Geometry: final body of the model. Coordinates: model frame, mm. A direction names the side the tool comes from. Give positions to 0.01 mm unless a question says otherwise; leave off trailing zeros. Write each loop counter-clockwise with the first axis right and the second up, starting at its lowest first coordinate (ties: lowest second). Pieces come first, ordered by that corner, then holes.
Q1. Line query: line 1 (Y direction, x = 0, z = 48.5); line 2 (X direction, y = -0.5, z = 54); line 3 (Z direction, x = -2, y = -1.5). Output: solid intervals per line, ascending.
Q2. Reachability of faces 4 (the flat face through (0, 0, 1.8)), 5 (the cylindrical face through (-4.336, -19.524, 41.961)), 6 (the flat face through (6.5, -3.86, 1)) from +Z, -Z, +X, -X, +Y, -Y: full face, straight path, thin tool, end or side. Return the list, or none.
Q3. Mould query, pull axis X, two halves, no side actions, for faces 1 (the cylindrical face through (-14.985, 0.66, 39.318)), 2 (the conical face through (15.446, 4.864, 0.194)), 3 (the flat face through (18, -6, 81)). Classes: +X half, -X half, draft (parallel to the pull), parting line (faces both ways), or undercut.
Q4. Pin query (flat end, axial travel): pin 1 Ø4 at (x, y) = (-14, -9.5) entering from -Z; pin 2 Ø12 at (x, z) = (-10.5, 60) entering from +Y; pin 3 Ø0.5 at (y, z) = (6, 0.5) entering from +X; pin 4 Ø10 at (y, z) = (-11, 46) entering from +X. Return the tip coordinate at first contact, or that it passes through.
Q5. Section A-A (z = 70). Return the cut outline in (x, y).
from build123d import *

# Parameters (mm, degrees)
F0_R      = 20
F1_DEPTH  = 81
F2_R      = 18.432207
F3_DEPTH  = 5.2
F4_R      = 15
F5_DEPTH  = 74
F6_SIZE   = 4
F7_R      = 1.125396
F8_DEPTH  = 1
F10_DEPTH = 1


with BuildPart() as f1:
    # F0 (on Top) → F1 (new body)
    with BuildSketch(Plane.XY):
        Circle(F0_R)
    extrude(amount=F1_DEPTH)

    # F2 (on face) → F3 (cut)
    with BuildSketch(Plane.XY.offset(81)):
        Circle(F2_R)
    extrude(amount=-F3_DEPTH, mode=Mode.SUBTRACT)

    # F4 (on face) → F5 (cut)
    with BuildSketch(Plane.XY.offset(75.8)):
        Circle(F4_R)
    extrude(amount=-F5_DEPTH, mode=Mode.SUBTRACT)

    # F6
    f6_edges = [f1.edges().sort_by_distance(p)[0] for p in [
        (-20, 0, 0),
    ]]
    chamfer(f6_edges, length=F6_SIZE)

    # F7 (on face) → F8 (cut)
    with BuildSketch(Plane(origin=(0, 0, 0), x_dir=(1, 0, 0), z_dir=(0, 0, -1))):
        Polygon((-6.869866, 12.288648), (-8.467419, 8.024589), (-3.123957, -5.726644), (0.010684, -5.726644), align=None)
        with Locations((-8.475489, -0.289656)):
            Circle(F7_R)
        Polygon((-11.636892, -2.851509), (-13.690377, -5.736166), (-10.554273, -5.736166), align=None)
    extrude(amount=-F8_DEPTH, mode=Mode.SUBTRACT)

    # F9 (on face) → F10 (cut)
    with BuildSketch(Plane(origin=(0, 0, 0), x_dir=(1, 0, 0), z_dir=(0, 0, -1))):
        with BuildLine():
            Line((5.370924, 12.654014), (-2.24095, 12.654014))
            Line((-2.24095, 12.654014), (-2.24095, 11.971393))
            Line((-2.24095, 11.971393), (5.390103, 11.971393))
            ThreePointArc((5.390103, 11.971393), (8.507735, 8.271818), (6.310662, 3.961442))
            Line((6.310662, 3.961442), (4.144951, 3.961442))
            Line((4.144951, 3.961442), (4.144951, 3.490261))
            Line((4.144951, 3.490261), (6.310662, 3.490261))
            ThreePointArc((6.310662, 3.490261), (9.895604, -0.9064), (7.034451, -5.804997))
            Line((7.034451, -5.804997), (6.007162, -5.804997))
            Line((6.007162, -5.804997), (6.007162, -6.437175))
            Line((6.007162, -6.437175), (7.073962, -6.437175))
            ThreePointArc((7.073962, -6.437175), (10.562571, -1.134228), (6.777628, 3.961442))
            ThreePointArc((6.777628, 3.961442), (9.053097, 8.789785), (5.370924, 12.654014))
        make_face()
    extrude(amount=-F10_DEPTH, mode=Mode.SUBTRACT)


solid = f1.part
Computed:
1. line 1: y = -20 to -15, 15 to 20
1. line 2: x = -19.99 to -14.99, 14.99 to 19.99
1. line 3: z = 0 to 1.8
2. face 4: +Z
2. face 5: +Z, -Z
2. face 6: -Z
3. face 1: undercut
3. face 2: parting line
3. face 3: draft
4. pin 1: stops at z = 0
4. pin 2: stops at y = 19.49
4. pin 3: stops at x = 15.65
4. pin 4: stops at x = 19.08
5. outline: circle Ø40 at (0, 0); hole circle Ø30 at (0, 0)
